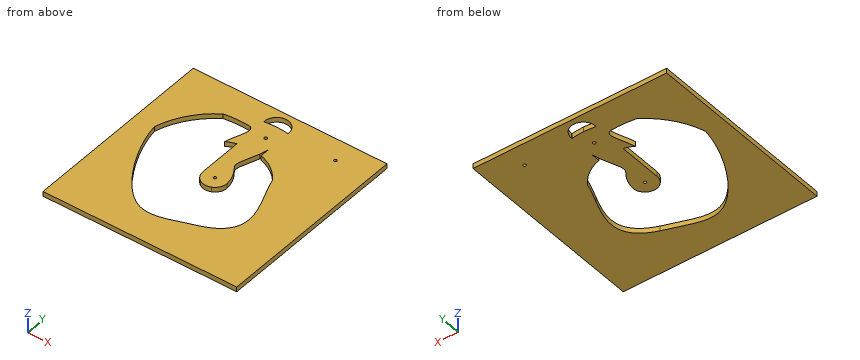
```python
from build123d import *

# Parameters (mm, degrees)
F0_W     = 200
F0_H     = 200
F1_DEPTH = 5
F2_R     = 1.5
F3_DEPTH = 5.001
F4_R     = 1.5
F5_DEPTH = 5.001


# Not quite as in the source:
# - a feature names something its author has since deleted; it is built from what else it names


with BuildPart() as f1:
    # F0 (on Top) → F1 (new body)
    with BuildSketch(Plane.XY):
        Rectangle(F0_W, F0_H)
    extrude(amount=F1_DEPTH)

    # F2 (on face) → F3 (cut, through all)
    with BuildSketch(Plane.XY.offset(5)):
        Circle(F2_R)
        with Locations((0, -63.662)):
            Circle(F2_R)
        with Locations((64.1583176089, 77.5462182691)):
            Circle(F2_R)
        with Locations((-51.9230208324, 31.0114389966)):
            Circle(F2_R)
        with Locations((1.6717778053, 65.3690844774)):
            Circle(F2_R)
    extrude(amount=-F3_DEPTH, mode=Mode.SUBTRACT)

    # F4 (on face) → F5 (cut, through all)
    with BuildSketch(Plane.XY.offset(5)):
        with BuildLine():
            Line((-12.5, 0), (-12.5, 45.3072841826))
            ThreePointArc((-12.5, 45.3072841826), (-17.4301226021, 43.6484916816), (-22.1467463119, 41.4550555156))
            add(Edge.make_bspline(
                [(-22.1467463119, 41.4550555156), (-22.9092474685, 38.6087716354), (-26.7916480004, 19.492616055), (-18.2157949408, -4.2593218119), (-6.9475647742, -10.3914072054)],
                knots=[0.382428707, 0.382428707, 0.382428707, 0.382428707, 0.4580536444, 0.8659002673, 0.8659002673, 0.8659002673, 0.8659002673], degree=3))
            ThreePointArc((-6.9475647742, -10.3914072054), (-11.024848291, -5.8909014727), (-12.5, 0))
        make_face()
        with BuildLine():
            ThreePointArc((-44.8138332434, 68.6711027291), (-66.3187168056, 48.2268369402), (-79.1399512645, 21.4678390587))
            add(Edge.make_bspline(
                [(28.4173693508, -56.6046871245), (3.9913801126, -64.1205269264), (-32.503865236, -87.7373972459), (-75.0211054276, -9.8932929428), (-79.1399512645, 21.4678390587)],
                knots=[0, 0, 0, 0, 0.2921661902, 0.6142842516, 0.6142842516, 0.6142842516, 0.6142842516], degree=3))
            add(Edge.make_bspline(
                [(28.4173693508, -56.6046871245), (64.8528327163, -43.3941669474), (56.1975225425, -18.4447190671), (46.7037719975, 5.2685558936)],
                knots=[0, 0, 0, 0, 0.1772966077, 0.1772966077, 0.1772966077, 0.1772966077], degree=3))
            ThreePointArc((46.7037719975, 5.2685558936), (46.9258845622, 2.6384385644), (47, 0))
            ThreePointArc((47, 0), (-24.1671566733, -40.310650433), (-22.1467463119, 41.4550555156))
            add(Edge.make_bspline(
                [(-18.0183753353, 69.6594335387), (-10.4657655575, 66.5625813654), (-18.2908445233, 55.8484646377), (-22.1467463119, 41.4550555156)],
                knots=[0, 0, 0, 0, 0.382428707, 0.382428707, 0.382428707, 0.382428707], degree=3))
            add(Edge.make_bspline(
                [(-44.8138332434, 68.6711027291), (-36.4977633391, 70.1220717043), (-27.3217936199, 70.3416004143), (-18.0183753353, 69.6594335387)],
                knots=[0.898151434, 0.898151434, 0.898151434, 0.898151434, 1, 1, 1, 1], degree=3))
        make_face()
        with Locations((0, -63.662)):
            Circle(F4_R, mode=Mode.SUBTRACT)
        with Locations((-51.9230208324, 31.0114389966)):
            Circle(F4_R, mode=Mode.SUBTRACT)
        with BuildLine():
            add(Edge.make_bspline(
                [(46.7037719975, 5.2685558936), (43.8279453898, 12.4517304214), (40.8751841388, 19.5214746733), (39.0755044059, 26.1171391125)],
                knots=[0.1772966077, 0.1772966077, 0.1772966077, 0.1772966077, 0.2310029169, 0.2310029169, 0.2310029169, 0.2310029169], degree=3))
            ThreePointArc((39.0755044059, 26.1171391125), (27.5149701187, 38.1041522589), (12.5, 45.3072841826))
            Line((12.5, 45.3072841826), (12.5, 0))
            ThreePointArc((12.5, 0), (10.548673601, -6.7063764627), (5.3039223586, -11.318940216))
            ThreePointArc((5.3039223586, -11.318940216), (-0.9436468985, -12.4643303282), (-6.9475647742, -10.3914072054))
            add(Edge.make_bspline(
                [(-22.1467463119, 41.4550555156), (-22.9092474685, 38.6087716354), (-26.7916480004, 19.492616055), (-18.2157949408, -4.2593218119), (-6.9475647742, -10.3914072054)],
                knots=[0.382428707, 0.382428707, 0.382428707, 0.382428707, 0.4580536444, 0.8659002673, 0.8659002673, 0.8659002673, 0.8659002673], degree=3))
            ThreePointArc((-22.1467463119, 41.4550555156), (-24.1671566733, -40.310650433), (47, 0))
            ThreePointArc((47, 0), (46.9258845622, 2.6384385644), (46.7037719975, 5.2685558936))
        make_face()
        with BuildLine():
            Line((12.5, 0), (12.5, 45.3072841826))
            ThreePointArc((12.5, 45.3072841826), (11.372638641, 45.6033232379), (10.2382828633, 45.8713152636))
            add(Edge.make_bspline(
                [(12.5, 0), (10.6902167617, 15.518115425), (-2.0681567086, 20.0495964199), (6.7073533039, 34.5490943361), (10.2382828633, 45.8713152636)],
                knots=[0, 0, 0, 0, 0.4638904895, 0.8993636987, 0.8993636987, 0.8993636987, 0.8993636987], degree=3))
        make_face()
        with BuildLine():
            Line((12.5, 45.3072841826), (12.5, 54.4343143702))
            add(Edge.make_bspline(
                [(10.2382828633, 45.8713152636), (11.0542680571, 48.4878400289), (11.8318981736, 51.3340910932), (12.5, 54.4343143702)],
                knots=[0.8993636987, 0.8993636987, 0.8993636987, 0.8993636987, 1, 1, 1, 1], degree=3))
            ThreePointArc((10.2382828633, 45.8713152636), (11.372638641, 45.6033232379), (12.5, 45.3072841826))
        make_face()
        with BuildLine():
            Line((-12.5, 82), (-12.5, 81.0416559554))
            ThreePointArc((-12.5, 81.0416559554), (-6.2683415531, 81.7600629536), (0, 82))
            ThreePointArc((0, 82), (6.2683415531, 81.7600629536), (12.5, 81.0416559554))
            Line((12.5, 81.0416559554), (12.5, 82))
            ThreePointArc((12.5, 82), (0, 94.5), (-12.5, 82))
        make_face()
    extrude(amount=-F5_DEPTH, mode=Mode.SUBTRACT)


solid = f1.part
```
Design review of the part built by this model. Coordinates are the model's own, in mm. Round coordinates to 2 decimals unless told otherwise and drop trailing zeros. Answer in a Markdown table with one row per item.
Q1. Clearance check with a flat-ended pin moving along its axis: pin 1 Ø1.8 at (x, y) = (0, 0) entering from +Z. State where the tip first meets the part, or that it passes through.
The answers:
| item | result |
|---|---|
| pin 1 | through |
Q2. Take a section at A-A, the plane y = 37. Count the separate pieces of the cut face and the enclosed holes in it, then the cut area to 3 significant figures.
The answers:
| item | result |
|---|---|
| separate pieces | 3 |
| enclosed holes | 0 |
| area | 587 mm² |
Q3. To check wall thickness, follow L1, parallel to Y at x = -8, z = 1.25; L2, parallel to X at y = -11, z = 2.45; L3, parallel to Y at x = -7, z = 4.55. State the ranges of each line that lie inside material, in increasing order. Write a range as [from, to].
The answers:
| item | result |
|---|---|
| L1 | [-100, -68.14], [-9.6, 81.61], [91.6, 100] |
| L2 | [-100, -69.97], [-5.94, 5.94], [52.55, 100] |
| L3 | [-100, -67.96], [-10.36, 81.7], [92.36, 100] |
